from build123d import *

# Parameters (mm, degrees)
BOSS_EXTRUDE1_DEPTH             = 15.875
BOSS_EXTRUDE1_DEPTH_BACK        = 15.875
SKETCH2_W                       = 330.2
SKETCH2_H                       = 9.525
F_1_4_0_25_DIAMETER_HOLE1_D     = 6.35
F_1_4_0_25_DIAMETER_HOLE1_DEPTH = 4.7625
F_1_4_0_25_DIAMETER_HOLE1_TIP   = 1.907732465


with BuildPart() as part:
    # Sketch2 → Boss-Extrude1 (new, two sides: drawn at the far end of the back side and taken through both)
    with BuildSketch(Plane(origin=(0, 0, 0), x_dir=(1, 0, 0), z_dir=(0, 1, 0)).offset(-BOSS_EXTRUDE1_DEPTH_BACK)):
        with Locations((0, 84.1375)):
            Rectangle(SKETCH2_W, SKETCH2_H)
    extrude(amount=BOSS_EXTRUDE1_DEPTH + BOSS_EXTRUDE1_DEPTH_BACK)

    # 1/4 (0.25) Diameter Hole1
    with Locations(Plane.XY.offset(-79.375)):
        with Locations((-142.875, 0), (-111.125, 0), (-79.375, 0), (-47.625, 0), (-15.875, 0), (15.875, 0), (47.625, 0), (79.375, 0), (111.125, 0), (142.875, 0)):
            Hole(F_1_4_0_25_DIAMETER_HOLE1_D / 2, depth=F_1_4_0_25_DIAMETER_HOLE1_DEPTH)
            with Locations((0, 0, -(F_1_4_0_25_DIAMETER_HOLE1_DEPTH + F_1_4_0_25_DIAMETER_HOLE1_TIP / 2))):  # 118° drill point
                Cone(0, F_1_4_0_25_DIAMETER_HOLE1_D / 2, F_1_4_0_25_DIAMETER_HOLE1_TIP, mode=Mode.SUBTRACT)


solid = part.part
The listing builds one solid part. Answer for the finished solid, in the listing's coordinates (mm). A direction names the side the tool comes from. Give positions to 0.01 mm unless a question says otherwise; leave off trailing zeros.
1) A tool of negligible diameter and unlimited length cuts with its end or side. For faces 5 (the face through (-2, 15.875, -84)), 6 (the face through (-82.403, 0.954, -81.79)), from which of +Z, -Z, +X, -X, +Y, -Y can it reach the whole face along a straight path? Write none if from no direction.
2) Section A-A (z = -81) is taken. Count the separate pieces of the cut face and the enclosed holes in it, and give its area (3 significant figures).
3) For a pull along Y with two mould halves and no side action, classify faces 1 (the face through (44.597, 0.954, -81.79)), 2 (the face through (-78.866, -0.211, -85.714)), 3 (the face through (-2, -15.875, -84)), 4 (the face through (-2, 0, -88.9)) as pulls with the +Y half, pulls with the -Y half, needs draft (parallel to the pull), parting line crosses it, or undercut.
4) Given P1, Ø5.5, axis at x = 142.875, y = 0, coming from the +Z side; P2, Ø5, axis at x = 47.625, y = 0, coming from the +Z side, each flat-ended and moving along its own axis, determine where each tip first touches the part or whether it passes through.
Response:
1. face 5: +Z, -Z, +X, -X, +Y
1. face 6: +Z
2. separate pieces: 1
2. enclosed holes: 10
2. area: 10,200 mm2
3. face 1: undercut
3. face 2: undercut
3. face 3: pulls with the -Y half
3. face 4: needs draft
4. P1: stops at z = -84.39
4. P2: stops at z = -84.54
